For this review, take the finished solid that the model builds, in its own axes (mm). Round coordinates to 2 decimals unless told otherwise and drop trailing zeros. Order: outer loops, then holes, each group sorted by start corner. A loop starts at its lowest first (then second) coordinate and runs counter-clockwise, first axis right, second up. Notation, with made-up numbers: (53.5, -2.5) - (88.5, -2.5) arc R22 ccw to (88.5, 6.5) - close; hole circle Ø5 at (11, -36.75). An arc over 180 degrees is marked (long way). Write each question's results on one line, items separated by ' | '. Start each with the question number.
(1) Take a section at D-D, the plane x = 76.5. Give the boundary of the cut face in (y, z), plus the area to 3 significant figures.
(2) Draft analysis for pull direction X (two halves, no side actions). For faces 1 (the cylindrical face through (52.23, 3.13, -1.04)), 2 (the flat face through (105, 3, 11)), 3 (the cylindrical face through (50.947, 3.219, -83.993)), 4 (the flat face through (51, 6.35, 10)), state which applies: pulls with the +X half, pulls with the -X half, needs draft (parallel to the pull), parting line crosses it, or undercut.
(3) Take a section at B-B, the plane y = 1.75. Give the number of separate pieces and of enclosed holes in the cut face, plus the area to 3 significant figures.
(4) Take a section at C-C, the plane z = -66. Give the boundary of the cut face in (x, y).
(5) Take a section at A-A, the plane x = 50. Give the boundary of the cut face in (y, z).
(6) For L1, parallel to X at y = 1.75, z = 67; L2, parallel to X at y = 4.25, z = -44; L3, parallel to X at y = 4.75, z = -10, list the stretches that pass through material, from the lowest coordinate up. Write a range as from..to.
```python
from build123d import *

# Parameters (mm, degrees)
SKETCH1_R           = 2.25
BOSS_EXTRUDE1_DEPTH = 6.35
SKETCH2_R           = 15
CUT_EXTRUDE1_DEPTH  = 10
CUT_EXTRUDE2_DEPTH  = 60
SKETCH4_R           = 2.25
CUT_EXTRUDE3_DEPTH  = 10


with BuildPart() as part:
    # Sketch1 → Boss-Extrude1 (new body)
    with BuildSketch(Plane(origin=(0, 0, 0), x_dir=(1, 0, 0), z_dir=(0, 1, 0))):
        Polygon((-5, -16), (-5, 84), (105, 84), (105, -16), (105, -71), (-5, -71), align=None)
        with Locations(Location((0, 0, 0), (0, 0, 270))):
            Circle(SKETCH1_R, mode=Mode.SUBTRACT)
        with Locations(Location((0, 44, 0), (0, 0, 270))):
            Circle(SKETCH1_R, mode=Mode.SUBTRACT)
        with Locations(Location((100, 44, 0), (0, 0, 270))):
            Circle(SKETCH1_R, mode=Mode.SUBTRACT)
        with Locations(Location((100, 0, 0), (0, 0, 270))):
            Circle(SKETCH1_R, mode=Mode.SUBTRACT)
        with Locations(Location((50, 43.25, 0), (0, 0, 270))):
            Circle(SKETCH1_R, mode=Mode.SUBTRACT)
        with Locations(Location((71.25, 22, 0), (0, 0, 270))):
            Circle(SKETCH1_R, mode=Mode.SUBTRACT)
        with Locations(Location((50, 0.75, 0), (0, 0, 270))):
            Circle(SKETCH1_R, mode=Mode.SUBTRACT)
        with Locations(Location((28.75, 22, 0), (0, 0, 270))):
            Circle(SKETCH1_R, mode=Mode.SUBTRACT)
    extrude(amount=BOSS_EXTRUDE1_DEPTH)

    # Sketch2 → Cut-Extrude1 (cut)
    with BuildSketch(Plane(origin=(0, 6.35, 0), x_dir=(1, 0, 0), z_dir=(0, 1, 0))):
        with Locations(Location((50, 22, 0), (0, 0, 270))):
            Circle(SKETCH2_R)
    extrude(amount=-CUT_EXTRUDE1_DEPTH, mode=Mode.SUBTRACT)

    # Sketch3 → Cut-Extrude2 (cut)
    with BuildSketch(Plane(origin=(0, 6.35, 0), x_dir=(1, 0, 0), z_dir=(0, 1, 0))):
        with BuildLine():
            Line((-11.87928751, 18.13298859), (-19.122468025, 134.037184903))
            Line((-19.122468025, 134.037184903), (176.364402691, 135.714155607))
            Line((176.364402691, 135.714155607), (111.227525883, 31.756540076))
            ThreePointArc((111.227525883, 31.756540076), (43.180433513, 83.623806381), (-11.87928751, 18.13298859))
        make_face()
    extrude(amount=-CUT_EXTRUDE2_DEPTH, mode=Mode.SUBTRACT)

    # Sketch4 → Cut-Extrude3 (cut)
    with BuildSketch(Plane.XZ):
        with Locations(Location((99.5, 67, 0), (0, 0, 270))):
            Circle(SKETCH4_R)
        with Locations(Location((0.5, 67, 0), (0, 0, 270))):
            Circle(SKETCH4_R)
        with Locations(Location((33.5, 67, 0), (0, 0, 270))):
            Circle(SKETCH4_R)
        with Locations(Location((66.5, 67, 0), (0, 0, 270))):
            Circle(SKETCH4_R)
    extrude(amount=-CUT_EXTRUDE3_DEPTH, mode=Mode.SUBTRACT)


solid = part.part
```
Results below:
1) outline: (0, -78.05) - (6.35, -78.05) - (6.35, 71) - (0, 71) - close | area: 946 mm^2
2) face 1: undercut | face 2: pulls with the +X half | face 3: parting line crosses it | face 4: needs draft
3) separate pieces: 1 | enclosed holes: 13 | area: 15,100 mm^2
4) outline: (6.32, 0) - (93.68, 0) - (93.68, 6.35) - (6.32, 6.35) - close
5) outline: (0, -84) - (6.35, -84) - (6.35, -45.5) - (0, -45.5) - close; (0, -41) - (6.35, -41) - (6.35, -37) - (0, -37) - close; (0, -7) - (6.35, -7) - (6.35, -3) - (0, -3) - close; (0, 1.5) - (6.35, 1.5) - (6.35, 71) - (0, 71) - close
6) L1: x = -5..-1.75, 2.75..31.25, 35.75..64.25, 68.75..97.25, 101.75..105 | L2: x = -5..-2.25, 2.25..47.88, 52.12..97.75, 102.25..105 | L3: x = -5..41, 59..105
